```python
from build123d import *

# Parameters (mm, degrees)
BOSS_EXTRUDE1_DEPTH = 15
SKETCH4_R           = 2.5
BOSS_EXTRUDE3_DEPTH = 5


with BuildPart() as part:
    # Sketch1 → Boss-Extrude1 (new body)
    with BuildSketch(Plane(origin=(0, 0, 0), x_dir=(0, 0, -1), z_dir=(1, 0, 0))):
        Polygon((0, 8.75), (1.617619032, 6.037036414), (4.375, 7.577722283), (4.419417382, 4.419417382), (7.577722283, 4.375), (6.037036414, 1.617619032), (8.75, 0), (6.037036414, -1.617619032), (7.577722283, -4.375), (4.419417382, -4.419417382), (4.375, -7.577722283), (1.617619032, -6.037036414), (0, -8.75), (-1.617619032, -6.037036414), (-4.375, -7.577722283), (-4.419417382, -4.419417382), (-7.577722283, -4.375), (-6.037036414, -1.617619032), (-8.75, 0), (-6.037036414, 1.617619032), (-7.577722283, 4.375), (-4.419417382, 4.419417382), (-4.375, 7.577722283), (-1.617619032, 6.037036414), align=None)
    boss_extrude1 = extrude(amount=BOSS_EXTRUDE1_DEPTH)

    # Sketch4 → Boss-Extrude3 (add)
    with BuildSketch(Plane(origin=(15, 0, 0), x_dir=(0, 0, -1), z_dir=(1, 0, 0))):
        Circle(SKETCH4_R)
    boss_extrude3 = extrude(amount=BOSS_EXTRUDE3_DEPTH)

    # Mirror1: Boss-Extrude1, Boss-Extrude3 across plane
    add(boss_extrude1.mirror(Plane(origin=(0, 0, 0), x_dir=(0, 0, 1), z_dir=(1, 0, 0))))
    add(boss_extrude3.mirror(Plane(origin=(0, 0, 0), x_dir=(0, 0, 1), z_dir=(1, 0, 0))))


solid = part.part
```
Verification items for the finished model (mm, model axes). A direction names the side the tool comes from. Round coordinates to 2 decimals unless told otherwise and drop trailing zeros. Write each loop counter-clockwise with the first axis right and the second up, starting at its lowest first coordinate (ties: lowest second). Pieces come first, ordered by that corner, then holes.
1. Draft check along Z on faces 6 (the cylindrical face through (17.46, -2.44, 0.54)), 7 (the flat face through (0.21, 6.82, 3.02)), 8 (the flat face through (-15, 2, -2)). Enter one of: +Z half, -Z half, draft (parallel to the pull), parting line (faces both ways), or undercut.
2. Section check C-C on y = 1. Enter the section's corners in (x, z), plus the area to 3 significant figures.
3. Section check D-D on z = -6.5. Enter the section's corners in (x, y), plus the area to 3 significant figures.
4. Scan lines: L1, parallel to Y at x = -5.5, z = 6.5; L2, parallel to Z at x = -10, y = 7; L3, parallel to Y at x = 10, z = 5. Record each from-to range of solid material in increasing order.
5. Section check B-B on x = 7. Enter the section's corners in (y, z) (3 decimals).
6. Access from +Z, -Z, +X, -X, +Y, -Y to the whole of each face (thin tool, end or side, straight path). Record for faces 1 (the cylindrical face through (-17.46, -2.44, 0.54)), 2 (the flat face through (0.21, -0.8, -7.41)), 3 (the flat face through (0.21, -6.82, -3.02)), 4 (the flat face through (0.21, -3.02, 6.82)), 5 (the flat face through (0.21, 6.8, -2.98)).
7. Section check A-A on z = 7. Enter the section's corners in (x, y).
8. Gauge pin test, flat ends, axial feed: P1, Ø5, axis at x = 0, z = 3, coming from the -Y side; P2, Ø3, axis at y = 4.5, z = 0.5, coming from the +X side; P3, Ø1.5, axis at y = 4.5, z = -4, coming from the -X side. Record the tip position at first contact, or that the pin passes through.
Answer:
1. face 6: parting line
1. face 7: undercut
1. face 8: draft
2. outline: (-20, -2.29) - (-15, -2.29) - (-15, -7.07) - (15, -7.07) - (15, -2.29) - (20, -2.29) - (20, 2.29) - (15, 2.29) - (15, 7.07) - (-15, 7.07) - (-15, 2.29) - (-20, 2.29) - close
2. area: 470 mm2
3. outline: (-15, -4.39) - (15, -4.39) - (15, -2.45) - (-15, -2.45) - close; (-15, -1.34) - (15, -1.34) - (15, 1.34) - (-15, 1.34) - close; (-15, 2.45) - (15, 2.45) - (15, 4.39) - (-15, 4.39) - close
3. area: 197 mm2
4. L1: y = -4.39 to -2.45, -1.34 to 1.34, 2.45 to 4.39
4. L2: z = -4.38 to -3.34, -1.04 to 1.04, 3.34 to 4.38
4. L3: y = -4.41 to 4.41
5. outline: (-8.75, 0) - (-6.037, -1.618) - (-7.578, -4.375) - (-4.419, -4.419) - (-4.375, -7.578) - (-1.618, -6.037) - (0, -8.75) - (1.618, -6.037) - (4.375, -7.578) - (4.419, -4.419) - (7.578, -4.375) - (6.037, -1.618) - (8.75, 0) - (6.037, 1.618) - (7.578, 4.375) - (4.419, 4.419) - (4.375, 7.578) - (1.618, 6.037) - (0, 8.75) - (-1.618, 6.037) - (-4.375, 7.578) - (-4.419, 4.419) - (-7.578, 4.375) - (-6.037, 1.618) - close
6. face 1: -X
6. face 2: -Z, +X, -X
6. face 3: +X, -X, -Y
6. face 4: +Z, +X, -X
6. face 5: +X, -X, +Y
7. outline: (-15, -4.38) - (15, -4.38) - (15, -3.34) - (-15, -3.34) - close; (-15, -1.04) - (15, -1.04) - (15, 1.04) - (-15, 1.04) - close; (-15, 3.34) - (15, 3.34) - (15, 4.38) - (-15, 4.38) - close
8. P1: stops at y = -7.91
8. P2: stops at x = 15
8. P3: stops at x = -15
